```python
from build123d import *

# Parameters (mm, degrees)
SKETCH_1_W          = 190
SKETCH_1_H          = 78
EXTRUDE_1_DEPTH     = 41
SKETCH_2_W          = 185
SKETCH_2_H          = 73
CUT_EXTRUDE_1_DEPTH = 38.5
SKETCH_3_W          = 2.5
SKETCH_3_H          = 73
CUT_EXTRUDE_2_DEPTH = 38.5
SKETCH_4_W          = 7
SKETCH_4_H          = 7
CUT_EXTRUDE_4_DEPTH = 2.5
SKETCH_5_W          = 10
SKETCH_5_H          = 4
CUT_EXTRUDE_5_DEPTH = 2.5
FILLET_1_R          = 1.5
SKETCH_9_W          = 15
SKETCH_9_H          = 2.5
CUT_EXTRUDE_8_DEPTH = 2.5
SKETCH_10_W         = 185
SKETCH_10_H         = 2.5
EXTRUDE_2_DEPTH     = 3
SKETCH_11_W         = 185
SKETCH_11_H         = 2.5
EXTRUDE_3_DEPTH     = 3
SKETCH_12_W         = 185
SKETCH_12_H         = 2.5
EXTRUDE_4_DEPTH     = 3
SKETCH_13_W         = 185
SKETCH_13_H         = 2.5
EXTRUDE_5_DEPTH     = 3


with BuildPart() as part:
    # 草图1 → 凸台-拉伸1 (new body)
    with BuildSketch(Plane(origin=(0, 0, 0), x_dir=(1, 0, 0), z_dir=(0, 1, 0))):
        with Locations((11.192771084, -10.259036145)):
            Rectangle(SKETCH_1_W, SKETCH_1_H)
    extrude(amount=EXTRUDE_1_DEPTH)

    # 草图2 → 切除-拉伸1 (cut)
    with BuildSketch(Plane(origin=(0, 41, 0), x_dir=(1, 0, 0), z_dir=(0, 1, 0))):
        with Locations((11.192771084, -10.259036145)):
            Rectangle(SKETCH_2_W, SKETCH_2_H)
    extrude(amount=-CUT_EXTRUDE_1_DEPTH, mode=Mode.SUBTRACT)

    # 草图3 → 切除-拉伸2 (cut)
    with BuildSketch(Plane(origin=(0, 41, 0), x_dir=(1, 0, 0), z_dir=(0, 1, 0))):
        with Locations((104.942771084, -10.259036145)):
            Rectangle(SKETCH_3_W, SKETCH_3_H)
    extrude(amount=-CUT_EXTRUDE_2_DEPTH, mode=Mode.SUBTRACT)

    # 草图4 → 切除-拉伸4 (cut)
    with BuildSketch(Plane.ZY.offset(83.807228916)):
        with Locations((-10.740963855, 23)):
            Rectangle(SKETCH_4_W, SKETCH_4_H)
        with Locations((33.059036145, 23)):
            Rectangle(SKETCH_4_W, SKETCH_4_H)
    extrude(amount=-CUT_EXTRUDE_4_DEPTH, mode=Mode.SUBTRACT)

    # 草图5 → 切除-拉伸5 (cut)
    with BuildSketch(Plane(origin=(0, 0, -28.740963855), x_dir=(-1, 0, 0), z_dir=(0, 0, -1))):
        with Locations((-44.692771084, 10.5)):
            Rectangle(SKETCH_5_W, SKETCH_5_H)
    extrude(amount=-CUT_EXTRUDE_5_DEPTH, mode=Mode.SUBTRACT)

    # 圆角1
    fillet_1_edges = [part.edges().sort_by_distance(p)[0] for p in [
        (39.692771084, 12.5, -27.490963855),
        (39.692771084, 8.5, -27.490963855),
        (49.692771084, 8.5, -27.490963855),
        (49.692771084, 12.5, -27.490963855),
    ]]
    fillet(fillet_1_edges, radius=FILLET_1_R)

    # 草图9 → 切除-拉伸8 (cut)
    with BuildSketch(Plane(origin=(-81.307228916, 0, 0), x_dir=(0, 0, -1), z_dir=(1, 0, 0))):
        with Locations((-29.259036145, 37.25)):
            Rectangle(SKETCH_9_W, SKETCH_9_H)
        with Locations((8.740963855, 37.25)):
            Rectangle(SKETCH_9_W, SKETCH_9_H)
    extrude(amount=-CUT_EXTRUDE_8_DEPTH, mode=Mode.SUBTRACT)

    # 草图10 → 凸台-拉伸2 (add)
    with BuildSketch(Plane(origin=(0, 0, 46.759036145), x_dir=(-1, 0, 0), z_dir=(0, 0, -1))):
        with Locations((-11.192771084, 39.75)):
            Rectangle(SKETCH_10_W, SKETCH_10_H)
    extrude(amount=EXTRUDE_2_DEPTH)

    # 草图11 → 凸台-拉伸3 (add)
    with BuildSketch(Plane.XY.offset(-26.240963855)):
        with Locations((11.192771084, 39.75)):
            Rectangle(SKETCH_11_W, SKETCH_11_H)
    extrude(amount=EXTRUDE_3_DEPTH)

    # 草图12 → 凸台-拉伸4 (add)
    with BuildSketch(Plane(origin=(0, 0, 46.759036145), x_dir=(-1, 0, 0), z_dir=(0, 0, -1))):
        with Locations((-11.192771084, 34.75)):
            Rectangle(SKETCH_12_W, SKETCH_12_H)
    extrude(amount=EXTRUDE_4_DEPTH)

    # 草图13 → 凸台-拉伸5 (add)
    with BuildSketch(Plane.XY.offset(-26.240963855)):
        with Locations((11.192771084, 34.75)):
            Rectangle(SKETCH_13_W, SKETCH_13_H)
    extrude(amount=EXTRUDE_5_DEPTH)


solid = part.part
```
Could you check a few things on this model? Use its own coordinates, in mm. A direction names the side the tool comes from. Coordinates: 2 decimals unless noted, no trailing zeros. Write each loop counter-clockwise with the first axis right and the second up, starting at its lowest first coordinate (ties: lowest second). Pieces come first, ordered by that corner, then holes. Notation, with made-up numbers: (31, 79.5) - (48, 79.5) arc R8 cw to (48, 91.5) - close; hole circle Ø2 at (65, -11.75). An arc over 180 degrees is marked (long way). Use a Markdown table: item, result.
Q1. Which directions (+Z, -Z, +X, -X, +Y, -Y) give clear straight access to the entire face, cutting with the end or side of a thin tool? Please do faces 1 (the flat face through (11, 18, -26.241)), 2 (the flat face through (10, 20, 49.259)).
Geometry check:
| item | result |
|---|---|
| face 1 | +X |
| face 2 | +Z, +X, -X, +Y, -Y |
Q2. Imagine slicing it at A-A (y = 21.5). List the corners of the cut face in (x, z) for me, and give its area (3 significant figures).
Geometry check:
| item | result |
|---|---|
| outline | (-83.81, -28.74) - (106.19, -28.74) - (106.19, -26.24) - (-81.31, -26.24) - (-81.31, -14.24) - (-83.81, -14.24) - close; (-83.81, -7.24) - (-81.31, -7.24) - (-81.31, 29.56) - (-83.81, 29.56) - close; (-83.81, 36.56) - (-81.31, 36.56) - (-81.31, 46.76) - (106.19, 46.76) - (106.19, 49.26) - (-83.81, 49.26) - close |
| area | 1,100 mm2 |
Q3. Imagine slicing it at C-C (x = 85.5). List the corners of the cut face in (y, z) for me, and give its area (4 significant figures).
Geometry check:
| item | result |
|---|---|
| outline | (0, -28.74) - (41, -28.74) - (41, -23.24) - (38.5, -23.24) - (38.5, -26.24) - (36, -26.24) - (36, -23.24) - (33.5, -23.24) - (33.5, -26.24) - (2.5, -26.24) - (2.5, 46.76) - (33.5, 46.76) - (33.5, 43.76) - (36, 43.76) - (36, 46.76) - (38.5, 46.76) - (38.5, 43.76) - (41, 43.76) - (41, 49.26) - (0, 49.26) - close |
| area | 417.5 mm2 |
Q4. Please list where these lines run through material, in increasing order: L1, parallel to Y at x = -7, z = 44; L2, parallel to Z at x = -5, y = 30; L3, parallel to Y at x = 54.5, z = -20.5.
Geometry check:
| item | result |
|---|---|
| L1 | y = 0 to 2.5, 33.5 to 36, 38.5 to 41 |
| L2 | z = -28.74 to -26.24, 46.76 to 49.26 |
| L3 | y = 0 to 2.5 |
Q5. Thinking about a two-plate mould opening in Z: for faces 3 (the flat face through (10, 20, -28.741)), 4 (the flat face through (11, 2.5, 10)), 5 (the flat face through (11, 18, 46.759)), 6 (the flat face through (12, 41, 45)), which applies, +Z half, -Z half, draft (parallel to the pull), parting line (faces both ways), or undercut?
Geometry check:
| item | result |
|---|---|
| face 3 | -Z half |
| face 4 | undercut |
| face 5 | undercut |
| face 6 | draft |
Q6. Imagine slicing it at B-B (z = -11). List the corners of the cut face in (x, y) for me, and give its area (4 significant figures).
Geometry check:
| item | result |
|---|---|
| outline | (-83.81, 0) - (106.19, 0) - (106.19, 2.5) - (-81.31, 2.5) - (-81.31, 19.5) - (-83.81, 19.5) - close; (-83.81, 26.5) - (-81.31, 26.5) - (-81.31, 36) - (-83.81, 36) - close; (-83.81, 38.5) - (-81.31, 38.5) - (-81.31, 41) - (-83.81, 41) - close |
| area | 547.5 mm2 |
Q7. I'm going to push flat-ended pins straight in: pin 1 Ø4 at (x, z) = (-61, -17) entering from +Y; pin 2 Ø1 at (y, z) = (13, 7.5) entering from +X; pin 3 Ø2 at (y, z) = (40.5, -25) entering from +X. Where does each tip first touch, or does it pass through?
Geometry check:
| item | result |
|---|---|
| pin 1 | stops at y = 2.5 |
| pin 2 | stops at x = -81.31 |
| pin 3 | stops at x = 103.69 |
Q8. Imagine slicing it at D-D (z = 12). List the corners of the cut face in (x, y) for me.
Geometry check:
| item | result |
|---|---|
| outline | (-83.81, 0) - (106.19, 0) - (106.19, 2.5) - (-81.31, 2.5) - (-81.31, 41) - (-83.81, 41) - close |
